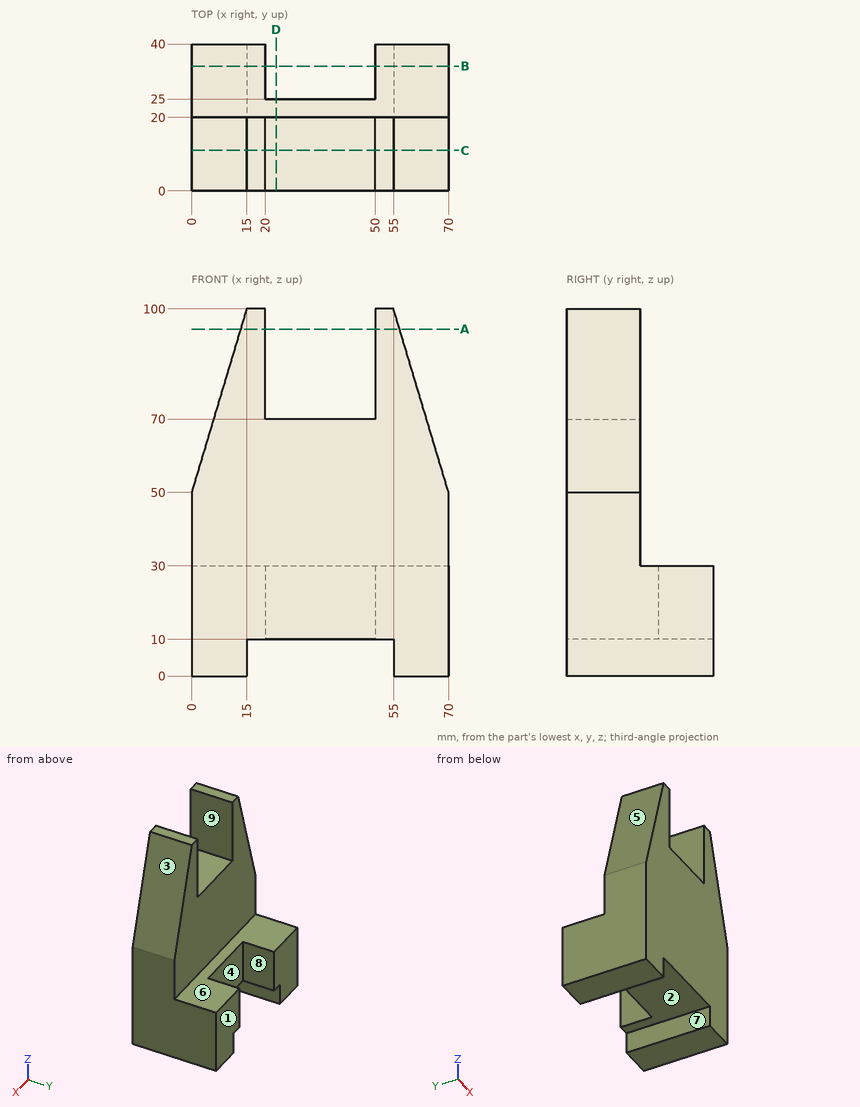
Can you work these out from the drawing? Everything is in mm from the part's minimum corner. A direction names the side the tool comes from. Coordinates: 2 decimals unless noted, no trailing zeros. Write each loop counter-clockwise with the first axis right and the second up, starting at its lowest first coordinate (ties: lowest second). Pieces come first, ordered by that corner, then holes. Notation, with made-up numbers: (-25, 52) - (23, 52) arc R19 cw to (23, 82) - close; hole circle Ø8 at (-24.5, 12). An arc over 180 degrees is marked (long way). One line per item, written item: value.
1) I need wall thicknesses on line 1 along Z through (x, y) = (65, 31.5); line 2 along Z through (x, y) = (19.5, 22); line 3 along X through (y, z) = (12, 73.5). Which ranges of each line are inside material? Lowest first, please.
Model answer:
line 1: z = 0 to 30
line 2: z = 10 to 30
line 3: x = 7.05 to 20, 50 to 62.95
2) Suppose I cut it at C-C on y = 11. Write out the boundary of the cut face in (x, z), and give its area (3 significant figures).
Model answer:
outline: (0, 0) - (15, 0) - (15, 10) - (55, 10) - (55, 0) - (70, 0) - (70, 50) - (55, 100) - (50, 100) - (50, 70) - (20, 70) - (20, 100) - (15, 100) - (0, 50) - close
area: 4,950 mm²
3) I'm going to push flat-ended pins straight in: P1, Ø2, axis at y = 22.5, z = 33, coming from the +X side; P2, Ø3, axis at y = 22.5, z = 3, coming from the -X side; P3, Ø22, axis at x = 33, y = 11.5, coming from the +Z side; P4, Ø22, axis at y = 7, z = 81, coming from the +X side. Where does each tip first touch, or does it pass through?
Model answer:
P1: passes through
P2: stops at x = 0
P3: stops at z = 70
P4: stops at x = 64
4) On a 3-axis mill with a long thin cutter (end or side, diameter ignored), from which of +Z, -Z, +X, -X, +Y, -Y can I reach the whole of each face in a straight line? I mean the marked faces 5, 6, 7, 8 and 9. Say none if no direction works.
Model answer:
face 5: +Z, -X, +Y, -Y
face 6: +Z, +X, -X, +Y
face 7: -Z, +Y, -Y
face 8: +Z, -Z, +Y
face 9: +Z, +Y, -Y
5) Suppose I cut it at A-A on z = 94.5. Write out the boundary of the cut face in (x, y), and give its area (3 significant figures).
Model answer:
outline: (13.35, 0) - (20, 0) - (20, 20) - (13.35, 20) - close; (50, 0) - (56.65, 0) - (56.65, 20) - (50, 20) - close
area: 266 mm²
6) Suppose I cut it at B-B on y = 34. Write out the boundary of the cut face in (x, z).
Model answer:
outline: (0, 0) - (15, 0) - (15, 10) - (20, 10) - (20, 30) - (0, 30) - close; (50, 10) - (55, 10) - (55, 0) - (70, 0) - (70, 30) - (50, 30) - close
7) We'd pull the mould along X, two halves only. Please class the marked faces 1, 2, 3 and 4: pulls with the +X half, pulls with the -X half, needs draft (parallel to the pull), parting line crosses it, or undercut.
Model answer:
face 1: needs draft
face 2: undercut
face 3: pulls with the +X half
face 4: undercut
8) Suppose I cut it at D-D on x = 23. Write out the boundary of the cut face in (y, z), and give its area (3 significant figures).
Model answer:
outline: (0, 10) - (25, 10) - (25, 30) - (20, 30) - (20, 70) - (0, 70) - close
area: 1,300 mm²
